Model file for the job. Use its own axes, mm. A direction names the side the tool comes from. Coordinates: 2 decimals unless noted, no trailing zeros. Write each loop counter-clockwise with the first axis right and the second up, starting at its lowest first coordinate (ties: lowest second). Pieces come first, ordered by that corner, then holes. Notation, with made-up numbers: M 46,34 L 69,34 A23 ccw 69,73 Z; hole C 39,25 d3. An arc over 180 degrees is marked long. One line per question, with ' | ' between items. Start each with the question number.
(1) Cut at C-C (z = 0.2). Write the cut outline in (x, y), plus the area to 3 significant figures.
(2) Tool access for faces 1 (the face through (6, 0, 1)), 2 (the face through (6.1, -0.85, 0.5)), 3 (the face through (6.1, 1.4, 0.5)), 4 (the face through (-1.335, -0.021, -0.197)): list every direction of +Z, -Z, +X, -X, +Y, -Y with a clear straight run to the whole face (end or side of a thin tool).
(3) Wall check: probe 1 along X at (y, z) = (1.8, 1.85); probe 2 along Z at (x, y) = (2.75, -1.55); probe 3 along Z at (x, y) = (3, 0.2). Give the ranges that are in metal, low to high.
(4) Two-plate mould, pull along X, no slides. Class faces 5 (the face through (1, 2.4, 1)), 6 (the face through (3.593, -0.143, -0.197)), 7 (the face through (6.74, 0.3, 0.5)): +X half, -X half, draft (parallel to the pull), parting line (faces both ways), or undercut.
(5) Flat gauge pins, fed straight in: pin 1 Ø1 at (x, y) = (6, 0) entering from +Z; pin 2 Ø0.8 at (x, z) = (6.5, 0.5) entering from +Y; pin 3 Ø1.4 at (x, y) = (-3.5, 0) entering from +Z. Where does each tip first touch, or does it go through?
(6) Cut at A-A (x = 3.14). Write the cut outline in (y, z) (3 decimals).
from build123d import *

# Parameters (mm, degrees)
F0_W     = 8.6
F0_H     = 4.8
F1_DEPTH = 3
F2_R     = 0.475
F3_DEPTH = 0.6
F4_SIZE  = 0.2
F5_W     = 1.3
F5_H     = 2.25
F6_DEPTH = 1
F7_W     = 1
F7_H     = 2.7
F8_DEPTH = 0.3
F9_R     = 0.29999


# Not quite as in the source:
# - a fillet or chamfer is up to 0.001 mm smaller than in the source, because OpenCascade refuses the exact size


with BuildPart() as f1:
    # F0 (on Top) → F1 (new body)
    with BuildSketch(Plane.XY):
        Rectangle(F0_W, F0_H)
    extrude(amount=F1_DEPTH)

    # F2 (on face) → F3 (join)
    with BuildSketch(Plane(origin=(0, 0, 0), x_dir=(1, 0, 0), z_dir=(0, 0, -1))):
        with Locations((-2, 0)):
            Circle(F2_R)
        with Locations((2, 0)):
            Circle(F2_R)
    extrude(amount=F3_DEPTH)

    # F4
    f4_edges = [f1.edges().sort_by_distance(p)[0] for p in [
        (-2.475, 0, -0.6),
        (1.525, 0, -0.6),
    ]]
    chamfer(f4_edges, length=F4_SIZE)

    # F5 (on Top) → F6 (join)
    with BuildSketch(Plane.XY):
        with Locations((-4.95, 0.275)):
            Rectangle(F5_W, F5_H)
        with Locations((4.95, 0.275)):
            Rectangle(F5_W, F5_H)
    extrude(amount=F6_DEPTH)

    # F7 (on face) → F8 (join)
    with BuildSketch(Plane.XY.offset(3)):
        with Locations((-1.14, 0)):
            Rectangle(F7_W, F7_H)
    extrude(amount=F8_DEPTH)

    # F9 (radius 0.3 in the source; OpenCascade refuses exactly that, so slightly less here)
    f9_edges = [f1.edges().sort_by_distance(p)[0] for p in [
        (-1.64, 0, 3.3),
        (-0.64, 0, 3.3),
    ]]
    fillet(f9_edges, radius=F9_R)


with BuildPart() as f1_1:
    # F10: moved
    add(f1.part.moved(Location((1.14, 0, 0))))


solid = f1_1.part
Filled in:
1) outline: M -4.46,-0.85 L -3.16,-0.85 L -3.16,-2.4 L 5.44,-2.4 L 5.44,-0.85 L 6.74,-0.85 L 6.74,1.4 L 5.44,1.4 L 5.44,2.4 L -3.16,2.4 L -3.16,1.4 L -4.46,1.4 Z | area: 47.1 mm²
2) face 1: +Z, +X, +Y, -Y | face 2: +Z, -Z, +X, -Y | face 3: +Z, -Z, +X, +Y | face 4: -Z
3) probe 1: -3.16 to 5.44 | probe 2: 0 to 3 | probe 3: -0.6 to 3
4) face 5: draft | face 6: undercut | face 7: +X half
5) pin 1: z = 1 | pin 2: y = 1.4 | pin 3: z = 3
6) outline: M -2.4,0 L -0.475,0 L -0.475,-0.4 L -0.275,-0.6 L 0.275,-0.6 L 0.475,-0.4 L 0.475,0 L 2.4,0 L 2.4,3 L -2.4,3 Z
